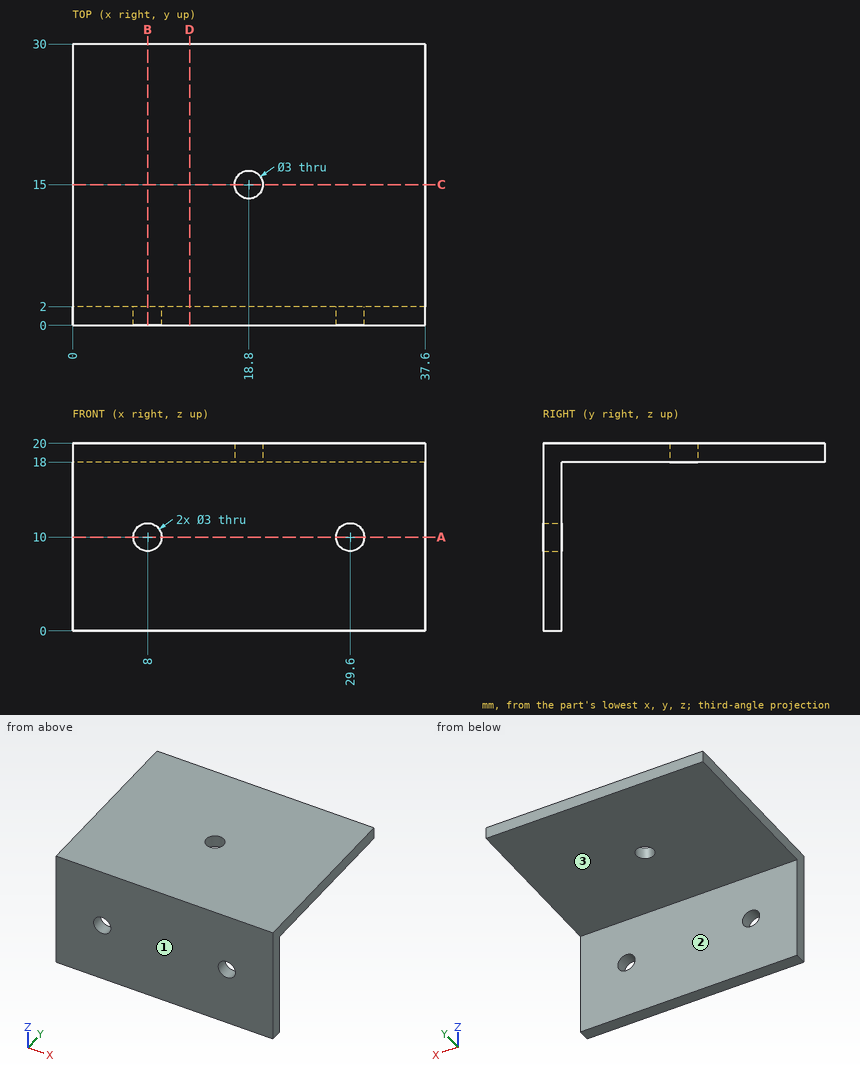
Verification items for this drawing (mm, ordinates from the low corner). Coordinates: 2 decimals unless noted, no trailing zeros. Order: outer loops, then holes, each group sorted by start corner. A loop starts at its lowest first (then second) coordinate and runs counter-clockwise, first axis right, second up.
Q1. Thickness scan on probe 1 along X at (y, z) = (0.9, 10); probe 2 along X at (y, z) = (15, 19.3); probe 3 along Z at (x, y) = (29.6, 1). Record the ranges inside material, lowest first.
Reply:
probe 1: x = 0 to 6.5, 9.5 to 28.1, 31.1 to 37.6
probe 2: x = 0 to 17.3, 20.3 to 37.6
probe 3: z = 0 to 8.5, 11.5 to 20
Q2. Sectioned sample at B-B on x = 8. Record the cut outline in (y, z).
Reply:
outline: (0, 0) - (2, 0) - (2, 8.5) - (0, 8.5) - close; (0, 11.5) - (2, 11.5) - (2, 18) - (30, 18) - (30, 20) - (0, 20) - close
Q3. Depth check by flat-ended pin: pin 1 Ø4 at (x, y) = (18.8, 15) entering from +Z; pin 2 Ø6 at (x, y) = (20, 23.5) entering from -Z; pin 3 Ø5 at (x, z) = (29.6, 10) entering from +Y. Enter the tip coordinate at first touch or a pass-through.
Reply:
pin 1: stops at z = 20
pin 2: stops at z = 18
pin 3: stops at y = 2
Q4. Sectioned sample at A-A on z = 10. Record the cut outline in (x, y), and give its area (3 significant figures).
Reply:
outline: (0, 0) - (6.5, 0) - (6.5, 2) - (0, 2) - close; (9.5, 0) - (28.1, 0) - (28.1, 2) - (9.5, 2) - close; (31.1, 0) - (37.6, 0) - (37.6, 2) - (31.1, 2) - close
area: 63.2 mm2
Q5. Sectioned sample at C-C on y = 15. Record the cut outline in (x, z).
Reply:
outline: (0, 18) - (17.3, 18) - (17.3, 20) - (0, 20) - close; (20.3, 18) - (37.6, 18) - (37.6, 20) - (20.3, 20) - close
Q6. Draft check along Y on the marked faces 1, 2 and 3. Enter one of: released by +Y, released by -Y, zero draft, split by the parting line, or undercut.
Reply:
face 1: released by -Y
face 2: released by +Y
face 3: zero draft
Q7. Sectioned sample at D-D on x = 12.5. Record the cut outline in (y, z).
Reply:
outline: (0, 0) - (2, 0) - (2, 18) - (30, 18) - (30, 20) - (0, 20) - close
